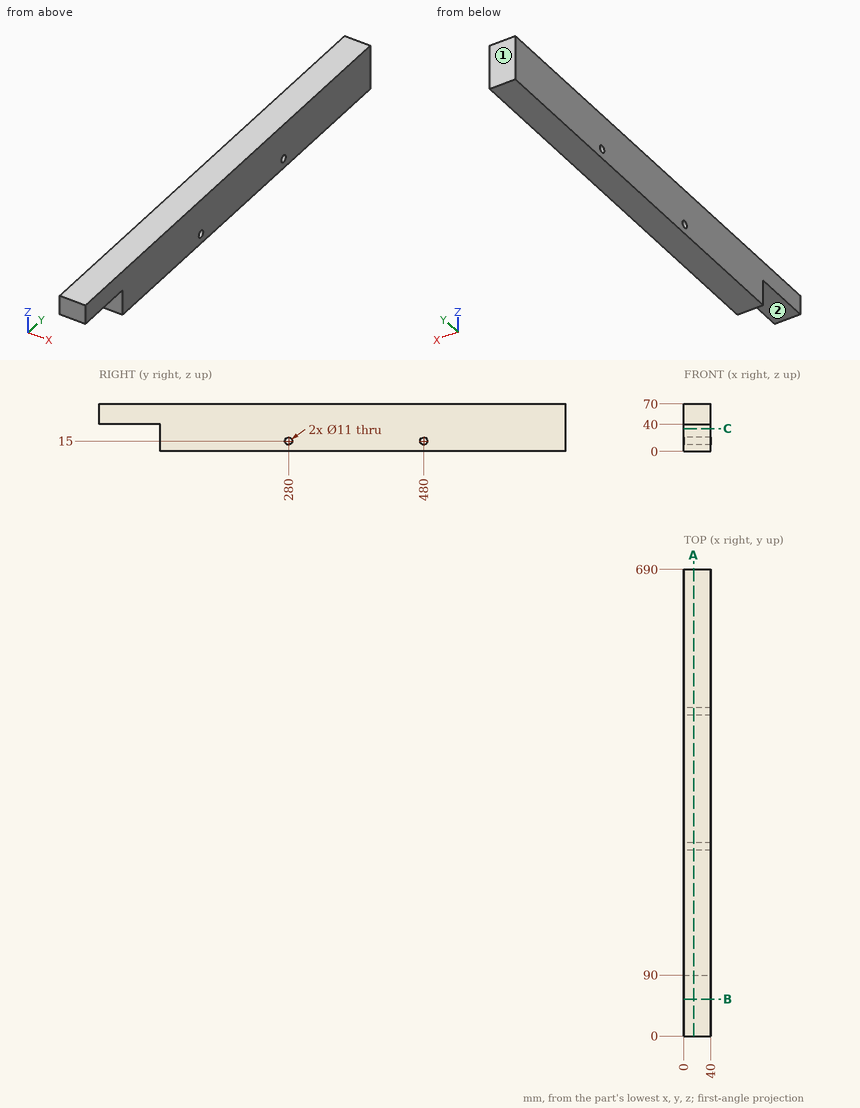
Here's the drawing with two shaded views (mm, measured from the low corner). I have some questions. A direction names the side the tool comes from. Give positions to 0.01 mm unless a question says otherwise; leave off trailing zeros. Order: outer loops, then holes, each group sorted by start corner. A loop starts at its lowest first (then second) coordinate and runs counter-clockwise, first axis right, second up. Notation, with made-up numbers: (-35, -16.75) -> (-9, -16.75) arc R13 cw to (-9, 4.25) -> close; hole circle Ø1 at (-17.75, 57.5). An arc over 180 degrees is marked (long way). Use a Markdown table: item, result. Add a question column.
Item 1: Imagine slicing it at B-B on y = 54.5. Please give me the cut outline in (x, z).
Item 2: Imagine slicing it at A-A on x = 14.5. Please give me the cut outline in (y, z).
Item 3: I need wall thicknesses on line 1 (Z direction, x = 21.5, y = 280); line 2 (Z direction, x = 30, y = 84); line 3 (Y direction, x = 18, z = 39.5). Which ranges of each line are inside material? Lowest first, please.
Item 4: Imagine slicing it at C-C on z = 33.5. Please give me the cut outline in (x, y).
Item 5: Will this pin go through, and if not, where does the flat tip stop? pin 1 (8 mm diameter, centred on x = 34.5, z = 30.5, fed in from -Y).
Item 6: For the marked faces 1 and 2, which set-ups out of +Z, -Z, +X, -X, +Y, -Y let a thin tool reach every point of the face, with its end or its side?
Data:
| question | item | result |
|---|---|---|
| 1 | outline | (0, 40) -> (40, 40) -> (40, 70) -> (0, 70) -> close |
| 2 | outline | (0, 40) -> (90, 40) -> (90, 0) -> (690, 0) -> (690, 70) -> (0, 70) -> close; hole circle Ø11 at (280, 15); hole circle Ø11 at (480, 15) |
| 3 | line 1 | z = 0 to 9.5, 20.5 to 70 |
| 3 | line 2 | z = 40 to 70 |
| 3 | line 3 | y = 90 to 690 |
| 4 | outline | (0, 90) -> (40, 90) -> (40, 690) -> (0, 690) -> close |
| 5 | pin 1 | stops at y = 90 |
| 6 | face 1 | +Z, -Z, +X, -X, +Y |
| 6 | face 2 | -Z, +X, -X, -Y |
